from build123d import *

# Parameters (mm, degrees)
F0_W     = 88.9
F0_H     = 38.1
F0_R     = 12.065
F1_DEPTH = 25.4
F2_W     = 88.9
F2_H     = 38.1
F3_DEPTH = 3.175


with BuildPart() as f1:
    # F0 (on Top) → F1 (new body)
    with BuildSketch(Plane.XY):
        with Locations((44.45, 19.05)):
            Rectangle(F0_W, F0_H)
        with Locations((19.05, 19.05)):
            Circle(F0_R, mode=Mode.SUBTRACT)
        with Locations((69.85, 19.05)):
            Circle(F0_R, mode=Mode.SUBTRACT)
    extrude(amount=F1_DEPTH)

    # F2 (on face) → F3 (join)
    with BuildSketch(Plane(origin=(0, 0, 0), x_dir=(1, 0, 0), z_dir=(0, 0, -1))):
        with Locations((44.45, -19.05)):
            Rectangle(F2_W, F2_H)
    extrude(amount=F3_DEPTH)


solid = f1.part
Design review of the part built by this model. Coordinates are the model's own, in mm. A direction names the side the tool comes from. Coordinates: 2 decimals unless noted, no trailing zeros. Order: outer loops, then holes, each group sorted by start corner. A loop starts at its lowest first (then second) coordinate and runs counter-clockwise, first axis right, second up. Notation, with made-up numbers: (76, 86) -> (127, 86) arc R24 cw to (127, 121) -> close; hole circle Ø3 at (-8.5, 79). An arc over 180 degrees is marked (long way). Use one line per item in the form item = value. Start each with the question number.
(1) The part is to be moulded in two halves that separate along Y. For faces 1 (the flat face through (44, 38.1, 11)), 2 (the flat face through (0, 19, 11)), 3 (the flat face through (19, 19, 0)), say which applies: +Y half, -Y half, draft (parallel to the pull), parting line (faces both ways), or undercut.
(2) Add section B-B on y = 19.05. State the section outline as (x, z) points (3 decimals), plus the area to 3 significant figures.
(3) Add section D-D on y = 15. State the section outline as (x, z) points (3 decimals), plus the area to 3 significant figures.
(4) Insertion check: pin 1 (7 mm diameter, centred on x = 17, y = 16, fed in from +Z). The pin has a flat end and moves straight along its axis. Give the tip position at first contact, or say it passes through.
(5) Add section A-A on z = 14.25. State the section outline as (x, y) points (3 decimals), plus the area to 3 significant figures.
(6) For probe 1 along Y at (x, z) = (19.05, 18) (3 decimals); probe 2 along X at (y, z) = (13, 20.25); probe 3 along X at (y, z) = (8, 24), list the stretches that pass through material, from the lowest coordinate up.
(7) Add section C-C on x = 69.85. State the section outline as (y, z) points (3 decimals), plus the area to 3 significant figures.
(8) For faces 4 (the flat face through (70, 19, 0)), 5 (the flat face through (44, 19, -3.175)), list the 3-axis set-ups (+Z, -Z, +X, -X, +Y, -Y) from which the entire face can be reached by the end or side of a thin tool; tool diameter is ignored.
Answer block:
q1.face_1 = +Y half
q1.face_2 = draft
q1.face_3 = undercut
q2.outline = (0, -3.175) -> (88.9, -3.175) -> (88.9, 25.4) -> (81.915, 25.4) -> (81.915, 0) -> (57.785, 0) -> (57.785, 25.4) -> (31.115, 25.4) -> (31.115, 0) -> (6.985, 0) -> (6.985, 25.4) -> (0, 25.4) -> close
q2.area = 1,310 mm²
q3.outline = (0, -3.175) -> (88.9, -3.175) -> (88.9, 25.4) -> (81.215, 25.4) -> (81.215, 0) -> (58.485, 0) -> (58.485, 25.4) -> (30.415, 25.4) -> (30.415, 0) -> (7.685, 0) -> (7.685, 25.4) -> (0, 25.4) -> close
q3.area = 1,390 mm²
q4.pin_1 = 0
q5.outline = (0, 0) -> (88.9, 0) -> (88.9, 38.1) -> (0, 38.1) -> close; hole circle Ø24.13 at (19.05, 19.05); hole circle Ø24.13 at (69.85, 19.05)
q5.area = 2,470 mm²
q6.probe_1 = 0 to 6.985, 31.115 to 38.1
q6.probe_2 = 0 to 8.61, 29.49 to 59.41, 80.29 to 88.9
q6.probe_3 = 0 to 14.21, 23.89 to 65.01, 74.69 to 88.9
q7.outline = (0, -3.175) -> (38.1, -3.175) -> (38.1, 25.4) -> (31.115, 25.4) -> (31.115, 0) -> (6.985, 0) -> (6.985, 25.4) -> (0, 25.4) -> close
q7.area = 476 mm²
q8.face_4 = +Z
q8.face_5 = -Z, +X, -X, +Y, -Y
